Autodesk Inventor part; units mm, degrees
ref_plane "YZ Plane" through (0, 0, 0) normal (1, 0, 0) x (0, 1, 0)
ref_plane "XZ Plane" through (0, 0, 0) normal (0, 1, 0) x (-1, 0, 0)
ref_plane "XY Plane" through (0, 0, 0) normal (0, 0, 1) x (1, 0, 0)
sketch "草图1" plane through (0, 0, 0) normal (1, 0, 0) x (0, 1, 0)
  point P0 (0, 0)
sketch "草图6" plane through (0, 0, 0) normal (1, 0, 0) x (0, 1, 0)
  line L0 (275, 0) -> (250, 15)
  line L1 (250, 15) -> (-250, 15)
  line L2 (-250, 15) -> (-275, 0)
  line L3 (-275, 0) -> (-250, -15)
  line L4 (-250, -15) -> (250, -15)
  line L5 (250, -15) -> (275, 0)
  point P0 (0, 0)
extrude "拉伸3" add sketch "草图6" along normal blind 300
properties part number "雪弗板"
Could you check a few things on this model? Use its own coordinates, in mm. Give positions to 0.01 mm unless a question says otherwise; leave off trailing zeros. Loops run counter-clockwise (first coordinate to the right, second up) from the corner with the lowest first, then second, coordinate; pieces in that order, holes last. Notation, with made-up numbers: (-22.5, -16.75) - (18.5, -16.75) arc R33 cw to (18.5, 14.25) - close; hole circle Ø4 at (16.25, 8). An arc over 180 degrees is marked (long way). Use one line per item in the form item = value.
1. I'm going to push a flat-ended pin straight in: pin 1 Ø4 at (x, z) = (232, 11.5) entering from -Y. Where does the tip first touch, or does it pass through?
Response values:
pin_1 = -259.17
2. I want a section at B-B (z = -5.75). Please give me the cut outline in (x, y).
Response values:
outline = (0, -265.42) - (300, -265.42) - (300, 265.42) - (0, 265.42) - close
3. I want a section at A-A (x = 121.5). Please give me the cut outline in (y, z), and give its area (4 significant figures).
Response values:
outline = (-275, 0) - (-250, -15) - (250, -15) - (275, 0) - (250, 15) - (-250, 15) - close
area = 15,750 mm²
4. I need wall thicknesses on probe 1 along Y at (x, z) = (206.5, 9.75); probe 2 along Y at (x, z) = (259, -7.5); probe 3 along Z at (x, y) = (42.5, -251). Which ranges of each line are inside material? Lowest first, please.
Response values:
probe_1 = -258.75 to 258.75
probe_2 = -262.5 to 262.5
probe_3 = -14.4 to 14.4
